Read the model definition and answer for the solid it produces. Units are mm, in the model's axes. A direction names the side the tool comes from. Coordinates: 2 decimals unless noted, no trailing zeros. Loops run counter-clockwise (first coordinate to the right, second up) from the corner with the lowest first, then second, coordinate; pieces in that order, holes last. Notation, with made-up numbers: (25.5, 4) -> (46.5, 4) arc R29 ccw to (46.5, 24) -> close; hole circle Ø9 at (25, 69.5). An arc over 180 degrees is marked (long way). Answer as a JSON object with one key per item and string values. Group by question number.
1) Section B-B, the plane y = -1 is taken. Give the vertices of the cut face in (x, z), plus the area to 3 significant figures.
2) Flat-ended cylindrical pins translate along their axes: P1, Ø3, axis at y = 9.5, z = 3, coming from the +X side (3 decimals); P2, Ø6, axis at x = 14, z = 14, coming from the -Y side; P3, Ø8, axis at y = 5.5, z = 7, coming from the +X side. Find the tip coordinate at first contact, or state that the pin passes through.
3) Section D-D, the plane x = 23.5 is taken. Give the vertices of the cut face in (y, z).
4) Section A-A, the plane x = 12 is taken. Give the vertices of the cut face in (y, z).
5) Determine the mould class of faces 3 (the face through (10.67, -7.796, 9.86)), 4 (the face through (16.59, 13.22, 9.86)), 5 (the face through (13.346, 0.629, 10.14)) for opening direction Y: released by +Y, released by -Y, zero draft, split by the parting line, or undercut.
6) Which of the six approach directions +Z, -Z, +X, -X, +Y, -Y give full straight-line access (tool end or side, diameter ignored) to faces 1 (the face through (15.342, 0.875, 10.14)), 2 (the face through (4.597, -2.117, 10.14))?
7) Section C-C, the plane z = 8 is taken. Give the vertices of the cut face in (x, y), plus the area to 3 significant figures.
8) Consider probe 1 along X at (y, z) = (3, 6.5); probe 2 along X at (y, z) = (0.25, 15.75); probe 3 along Y at (x, z) = (8.5, 17). Determine where each line is inside the solid, lowest interval first. Write a range as [from, to].
from build123d import *

# Parameters (mm, degrees)
BOSS_EXTRU_1_DEPTH      = 20
ENL_V_MAT_EXTRU_1_DEPTH = 20
ENL_V_MAT_EXTRU_2_DEPTH = 20


with BuildPart() as part:
    # Esquisse1 → Boss.-Extru.1 (new body)
    with BuildSketch(Plane.XY):
        Polygon((0, 0), (10.591231248, 16.965430164), (27.556661412, 6.374198916), (29.810281051, -3.368552159), (2.257780804, -9.74178761), align=None)
    extrude(amount=BOSS_EXTRU_1_DEPTH)

    # Esquisse3 → Enlèv. mat.-Extru.1 (cut)
    with BuildSketch(Plane.XY.offset(20)):
        Polygon((15.059755827, -6.780531881), (17.008306042, -6.329807952), (13.627876577, 8.28431866), (11.679326362, 7.833594731), align=None)
    extrude(amount=-ENL_V_MAT_EXTRU_1_DEPTH, mode=Mode.SUBTRACT)

    # Esquisse4 → Enlèv. mat.-Extru.2 (cut)
    with BuildSketch(Plane.XY.offset(20)):
        Polygon((6.154881268, -8.8403399), (2.994373603, 4.796499582), (-5.37239396, 2.5559716), (0.883083606, -10.672172042), (6.394810123, -10.300296517), align=None)
        Polygon((25.913180592, -4.269999889), (22.758113126, 9.369851491), (37.693290305, 8.113830617), (39.464159746, -8.899165087), (30.389447251, -4.288402222), align=None)
    extrude(amount=-ENL_V_MAT_EXTRU_2_DEPTH, mode=Mode.SUBTRACT)


solid = part.part
Determined:
{
 "1": {"outline": "(4.34, 0) -> (13.72, 0) -> (13.72, 20) -> (4.34, 20) -> close; (15.78, 0) -> (25.16, 0) -> (25.16, 20) -> (15.78, 20) -> close", "area": "375 mm²"},
 "2": {"P1": "x = 23.075", "P2": "y = -7.72", "P3": "x = 24.58"},
 "3": {"outline": "(-4.83, 0) -> (6.16, 0) -> (6.16, 20) -> (-4.83, 20) -> close"},
 "4": {"outline": "(-7.49, 0) -> (6.45, 0) -> (6.45, 20) -> (-7.49, 20) -> close; (7.91, 0) -> (16.09, 0) -> (16.09, 20) -> (7.91, 20) -> close"},
 "5": {"face 3": "released by -Y", "face 4": "released by +Y", "face 5": "undercut"},
 "6": {"face 1": "+Z, -Z", "face 2": "+Z, -Z, -X, -Y"},
 "7": {"outline": "(2.99, 4.8) -> (6.15, -8.84) -> (15.06, -6.78) -> (11.68, 7.83) -> (13.63, 8.28) -> (17.01, -6.33) -> (25.91, -4.27) -> (22.76, 9.37) -> (10.59, 16.97) -> close", "area": "357 mm²"},
 "8": {"probe 1": "[3.41, 12.8], [14.85, 24.23]", "probe 2": "[4.05, 13.43], [15.49, 24.87]", "probe 3": "[-8.3, 13.62]"}
}
